```python
from build123d import *

# Parameters (mm, degrees)
SKETCH1_W           = 260
SKETCH1_H           = 85
BOSS_EXTRUDE1_DEPTH = 2.5
SKETCH2_W           = 85
SKETCH2_H           = 260
SKETCH2_W_2         = 80
SKETCH2_H_2         = 255
BOSS_EXTRUDE2_DEPTH = 35
SKETCH3_W           = 85
SKETCH3_H           = 260
BOSS_EXTRUDE3_DEPTH = 6
SKETCH4_W           = 260
SKETCH4_H           = 43.5
CUT_EXTRUDE1_DEPTH  = 2.5
CUT_EXTRUDE2_REACH  = 45.5
SKETCH5_W           = 8.5
SKETCH5_H           = 16
SKETCH14_R          = 8.25
CUT_EXTRUDE8_DEPTH  = 2.5
SKETCH22_R          = 8.25
CUT_EXTRUDE9_DEPTH  = 10
CUT_EXTRUDE11_REACH = 45.5
SKETCH25_W          = 20.88469263
SKETCH25_H          = 3.5
SKETCH27_W          = 30
SKETCH27_H          = 43.5
BOSS_EXTRUDE4_DEPTH = 2.5
SKETCH29_W          = 2.5
SKETCH29_H          = 20
BOSS_EXTRUDE5_DEPTH = 10
SKETCH30_W          = 6
SKETCH30_H          = 20
CUT_EXTRUDE12_DEPTH = 5


with BuildPart() as part:
    # Sketch1 → Boss-Extrude1 (new body)
    with BuildSketch(Plane(origin=(0, 0, 0), x_dir=(0, 1, 0), z_dir=(0, 0, 1))):
        Rectangle(SKETCH1_W, SKETCH1_H)
    extrude(amount=BOSS_EXTRUDE1_DEPTH)

    # Sketch2 → Boss-Extrude2 (add)
    with BuildSketch(Plane(origin=(0, 0, 0), x_dir=(1, 0, 0), z_dir=(0, 0, -1))):
        Rectangle(SKETCH2_W, SKETCH2_H)
        Rectangle(SKETCH2_W_2, SKETCH2_H_2, mode=Mode.SUBTRACT)
    extrude(amount=BOSS_EXTRUDE2_DEPTH)

    # Sketch3 → Boss-Extrude3 (add)
    with BuildSketch(Plane(origin=(0, 0, -35), x_dir=(1, 0, 0), z_dir=(0, 0, -1))):
        Rectangle(SKETCH3_W, SKETCH3_H)
    extrude(amount=BOSS_EXTRUDE3_DEPTH)

    # Sketch4 → Cut-Extrude1 (cut)
    with BuildSketch(Plane(origin=(-42.5, 0, 0), x_dir=(0, -1, 0), z_dir=(-1, 0, 0))):
        with Locations((0, -19.25)):
            Rectangle(SKETCH4_W, SKETCH4_H)
    extrude(amount=-CUT_EXTRUDE1_DEPTH, mode=Mode.SUBTRACT)

    # Sketch5 → Cut-Extrude2 (cut, up to next)
    with BuildSketch(Plane.XY.offset(2.5), mode=Mode.PRIVATE) as cut_extrude2_sk1:
        with Locations((-33.25, 0)):
            Rectangle(SKETCH5_W, SKETCH5_H)
    cut_extrude2_tool1 = extrude(cut_extrude2_sk1.sketch, amount=-CUT_EXTRUDE2_REACH, mode=Mode.PRIVATE) & part.part
    add(cut_extrude2_tool1.solids().sort_by_distance((-33.25, 0, 2.5))[0], mode=Mode.SUBTRACT)

    # Sketch14 → Cut-Extrude8 (cut)
    with BuildSketch(Plane.XZ.offset(130)):
        with Locations((-20.95492543, -21.33509917)):
            Circle(SKETCH14_R)
    extrude(amount=-CUT_EXTRUDE8_DEPTH, mode=Mode.SUBTRACT)

    # Sketch22 → Cut-Extrude9 (cut)
    with BuildSketch(Plane(origin=(0, 130, 0), x_dir=(-1, 0, 0), z_dir=(0, 1, 0))):
        with Locations((-24.702923979, -21.634364917)):
            Circle(SKETCH22_R)
        with Locations((-2.202923979, -21.634364917)):
            Circle(SKETCH22_R)
        with Locations((20.297076021, -21.634364917)):
            Circle(SKETCH22_R)
    extrude(amount=-CUT_EXTRUDE9_DEPTH, mode=Mode.SUBTRACT)

    # Sketch25 → Cut-Extrude11 (cut, up to next)
    with BuildSketch(Plane.XY.offset(2.5), mode=Mode.PRIVATE) as cut_extrude11_sk1:
        with Locations((24.557653685, -121.75)):
            Rectangle(SKETCH25_W, SKETCH25_H)
    cut_extrude11_tool1 = extrude(cut_extrude11_sk1.sketch, amount=-CUT_EXTRUDE11_REACH, mode=Mode.PRIVATE) & part.part
    add(cut_extrude11_tool1.solids().sort_by_distance((24.557654, -121.75, 2.5))[0], mode=Mode.SUBTRACT)

    # Sketch27 → Boss-Extrude4 (add)
    with BuildSketch(Plane(origin=(-40, 0, 0), x_dir=(0, -1, 0), z_dir=(-1, 0, 0))):
        with Locations((-115, -19.25)):
            Rectangle(SKETCH27_W, SKETCH27_H)
        with Locations((115, -19.25)):
            Rectangle(SKETCH27_W, SKETCH27_H)
    extrude(amount=-BOSS_EXTRUDE4_DEPTH)

    # Sketch29 → Boss-Extrude5 (add)
    with BuildSketch(Plane.XY.offset(2.5)):
        with Locations((26.25, -105)):
            Rectangle(SKETCH29_W, SKETCH29_H)
    boss_extrude5 = extrude(amount=BOSS_EXTRUDE5_DEPTH)

    # Sketch30 → Cut-Extrude12 (cut)
    with BuildSketch(Plane.XY.offset(2.5)):
        with Locations((22, -105)):
            Rectangle(SKETCH30_W, SKETCH30_H)
    cut_extrude12 = extrude(amount=-CUT_EXTRUDE12_DEPTH, mode=Mode.SUBTRACT)

    # Mirror2: Boss-Extrude5, Cut-Extrude12 across plane
    add(boss_extrude5.mirror(Plane.ZX))
    add(cut_extrude12.mirror(Plane.ZX), mode=Mode.SUBTRACT)


solid = part.part
```
Work out the finished part from the listing and answer in its coordinate system (mm). A direction names the side the tool comes from. Round coordinates to 2 decimals unless told otherwise and drop trailing zeros. Loops run counter-clockwise (first coordinate to the right, second up) from the corner with the lowest first, then second, coordinate; pieces in that order, holes last. Notation, with made-up numbers: (-19.5, 57) -> (-13.5, 57) arc R31 ccw to (-13.5, 88) -> close; hole circle Ø5 at (43.25, 34.5). An arc over 180 degrees is marked (long way). Write each question's results on one line, items separated by ' | '. Start each with the question number.
1. A tool of negligible diameter and unlimited length cuts with its end or side. For faces 4 (the face through (-1, -2, 0)), 5 (the face through (-2.232, 128.768, -14.678)), 6 (the face through (27.5, -105, 7)), from which of +Z, -Z, +X, -X, +Y, -Y can it reach the whole face along a straight path? Write none if from no direction.
2. Section A-A (z = -18) is taken. Determine the outline of the cut face in (x, y), plus the area to 3 significant figures.
3. Find the intervals of material crossed by probe 1 along Y at (x, z) = (34.5, -1.5); probe 2 along Z at (x, y) = (-25, -11); probe 3 along X at (y, z) = (-111, -13.5), in increasing order. Write a range as from..to.
4. For a pull along Y with two mould halves and no side action, classify faces 1 (the face through (-14.216, 128.768, -16.059)), 2 (the face through (1, -127.5, -17)), 3 (the face through (1, -130, -19)) as +Y half, -Y half, draft (parallel to the pull), parting line (faces both ways), or undercut.
5. Section B-B (x = -17) is taken. Determine the outline of the cut face in (y, z).
6. Section C-C (y = 12.5) is taken. Determine the outline of the cut face in (x, z), plus the area to 3 significant figures.
7. Given pin 1 Ø0.8 at (x, z) = (26.5, 5) entering from -Y; pin 2 Ø6 at (x, y) = (4, 70.5) entering from +Z; pin 3 Ø19 at (x, z) = (-20.95, -21.34) entering from +Y, each flat-ended and moving along its own axis, determine where each tip first touches the part or whether it passes through.
8. Section D-D (x = 3) is taken. Determine the outline of the cut face in (y, z).
Evaluation:
1) face 4: none | face 5: +Y | face 6: +Z, +X, +Y, -Y
2) outline: (-40, -130) -> (-28.5, -130) -> (-28.5, -127.5) -> (-37.5, -127.5) -> (-37.5, -100) -> (-40, -100) -> close; (-40, 100) -> (-37.5, 100) -> (-37.5, 127.5) -> (-27.7, 127.5) -> (-27.7, 130) -> (-40, 130) -> close; (-13.41, -130) -> (42.5, -130) -> (42.5, 130) -> (32.11, 130) -> (32.11, 127.5) -> (40, 127.5) -> (40, -127.5) -> (-13.41, -127.5) -> close; (-12.89, 127.5) -> (-5.2, 127.5) -> (-5.2, 130) -> (-12.89, 130) -> close; (9.61, 127.5) -> (17.3, 127.5) -> (17.3, 130) -> (9.61, 130) -> close | area: 1,040 mm2
3) probe 1: y = -130..-127.5, 127.5..130 | probe 2: z = -41..-35, 0..2.5 | probe 3: x = -40..-37.5, 40..42.5
4) face 1: draft | face 2: undercut | face 3: -Y half
5) outline: (-130, -41) -> (130, -41) -> (130, -29.2) -> (127.5, -29.2) -> (127.5, -35) -> (-127.5, -35) -> (-127.5, -28.58) -> (-130, -28.58) -> close; (-130, -14.09) -> (-127.5, -14.09) -> (-127.5, 0) -> (127.5, 0) -> (127.5, -14.07) -> (130, -14.07) -> (130, 2.5) -> (-130, 2.5) -> close
6) outline: (-40, -41) -> (42.5, -41) -> (42.5, 2.5) -> (-40, 2.5) -> (-40, 0) -> (40, 0) -> (40, -35) -> (-40, -35) -> close | area: 789 mm2
7) pin 1: stops at y = -115 | pin 2: stops at z = 2.5 | pin 3: stops at y = 130
8) outline: (-130, -41) -> (130, -41) -> (130, -29.85) -> (127.5, -29.85) -> (127.5, -35) -> (-127.5, -35) -> (-127.5, 0) -> (127.5, 0) -> (127.5, -13.42) -> (130, -13.42) -> (130, 2.5) -> (-130, 2.5) -> close
